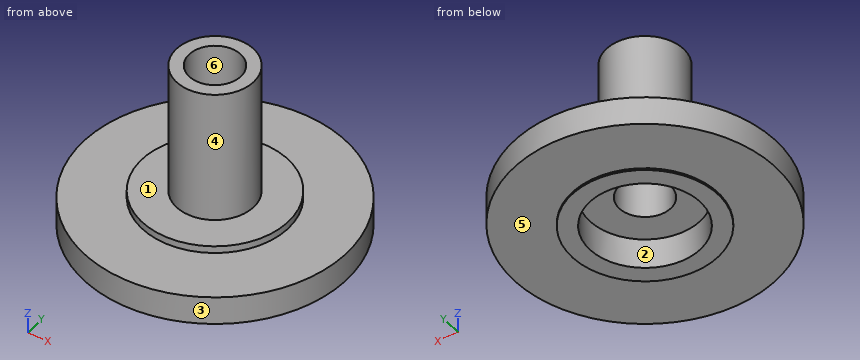
```python
from build123d import *

# Parameters (mm, degrees)
F0_R     = 2.6162
F0_R_2   = 1.75
F1_DEPTH = 9.52
F0_R_3   = 4.950253
F0_R_4   = 3.75
F2_DEPTH = 0.4826
F3_DEPTH = 2.05
F0_R_5   = 8.89
F4_DEPTH = 1.92


with BuildPart() as f1:
    # F0 (on Top) → F1 (new body)
    with BuildSketch(Plane.XY):
        Circle(F0_R)
        Circle(F0_R_2, mode=Mode.SUBTRACT)
    extrude(amount=F1_DEPTH)

    # F0 (on Top) → F2 (join)
    with BuildSketch(Plane.XY):
        Circle(F0_R_3)
        Circle(F0_R_4, mode=Mode.SUBTRACT)
        Circle(F0_R_4)
        Circle(F0_R, mode=Mode.SUBTRACT)
    extrude(amount=F2_DEPTH)

    # F0 (on Top) → F3 (join)
    with BuildSketch(Plane.XY):
        Circle(F0_R_3)
        Circle(F0_R_4, mode=Mode.SUBTRACT)
    extrude(amount=-F3_DEPTH)

    # F0 (on Top) → F4 (join)
    with BuildSketch(Plane.XY):
        Circle(F0_R_5)
        Circle(F0_R_3, mode=Mode.SUBTRACT)
    extrude(amount=-F4_DEPTH)


solid = f1.part
```
Could you check a few things on this model? Use its own coordinates, in mm. Face numbers are marked on the shaded views. A direction names the side the tool comes from. Give positions to 0.01 mm unless a question says otherwise; leave off trailing zeros. Order: outer loops, then holes, each group sorted by start corner. A loop starts at its lowest first (then second) coordinate and runs counter-clockwise, first axis right, second up.
Q1. Suppose I cut it at A-A, the plane x = 0. Write out the boundary of the cut face in (y, z), and give its area (3 significant figures).
Q2. If I drill on line 1 along Y through (x, z) = (0, 5.5); line 2 along Z through (x, y) = (1, 1.75); line 3 along Z through (x, y) = (-4, -3), over which ranges is the centre line in solid material (lowest first)?
Q3. Suppose I cut it at C-C, the plane z = 0.25. Write out the boundary of the cut face in (x, y), and give its area (3 significant figures).
Q4. For the marked faces 1, 2 and 3, which set-ups out of +Z, -Z, +X, -X, +Y, -Y let a thin tool reach every point of the face, with its end or its side?
Q5. We'd pull the mould along Y, two halves only. Please class the marked faces 4, 5 and 6: +Y half, -Y half, draft (parallel to the pull), parting line (faces both ways), or undercut.
Q6. I'm going to push flat-ended pins straight in: P1, Ø4.5, axis at x = 0, y = 0, coming from the -Z side; P2, Ø1.5, axis at x = 7, y = 0, coming from the -Z side; P3, Ø6, axis at y = 3.5, z = 2, coming from the -X side. Where does each tip first touch, or does it pass through?
Q7. Suppose I cut it at D-D, the plane y = -3. Write out the boundary of the cut face in (x, z), and give its area (3 significant figures).
Solution:
1. outline: (-8.89, -1.92) - (-4.95, -1.92) - (-4.95, -2.05) - (-3.75, -2.05) - (-3.75, 0) - (-1.75, 0) - (-1.75, 9.52) - (-2.62, 9.52) - (-2.62, 0.48) - (-4.95, 0.48) - (-4.95, 0) - (-8.89, 0) - close; (1.75, 0) - (3.75, 0) - (3.75, -2.05) - (4.95, -2.05) - (4.95, -1.92) - (8.89, -1.92) - (8.89, 0) - (4.95, 0) - (4.95, 0.48) - (2.62, 0.48) - (2.62, 9.52) - (1.75, 9.52) - close
1. area: 38.8 mm2
2. line 1: y = -2.62 to -1.75, 1.75 to 2.62
2. line 2: z = 0 to 9.52
2. line 3: z = -1.92 to 0
3. outline: circle Ø9.9 at (0, 0); hole circle Ø3.5 at (0, 0)
3. area: 67.4 mm2
4. face 1: +Z
4. face 2: -Z
4. face 3: +Z, -Z
5. face 4: parting line
5. face 5: draft
5. face 6: undercut
6. P1: stops at z = 0
6. P2: stops at z = -1.92
6. P3: stops at x = -8.8
7. outline: (-8.37, -1.92) - (-3.94, -1.92) - (-3.94, -2.05) - (-2.25, -2.05) - (-2.25, 0) - (2.25, 0) - (2.25, -2.05) - (3.94, -2.05) - (3.94, -1.92) - (8.37, -1.92) - (8.37, 0) - (3.94, 0) - (3.94, 0.48) - (-3.94, 0.48) - (-3.94, 0) - (-8.37, 0) - close
7. area: 27.7 mm2
